```python
from build123d import *

# Parameters (mm, degrees)
F2_DEPTH = 105.9625
F3_W     = 176.60625
F3_H     = 3
F4_DEPTH = 6.35
F5_W     = 176.60625
F5_H     = 3
F6_DEPTH = 6.35


# Not quite as in the source:
# - a length typed as a fraction of an inch, garbled in the dataset ("3 / 203.2 mm" for 3/8 in), is restored


with BuildPart() as f2:
    # F1 (on Front) → F2 (new body)
    with BuildSketch(Plane.XZ):
        Polygon((-42.2606132925, -1.7798869123), (-42.2606132925, -4.7798869123), (134.3456367075, -4.7798869123), (134.3456367075, -1.7798869123), (127.9956367075, -1.7798869123), (127.9956367075, 1.2201130877), (-35.9106132925, 1.2201130877), (-35.9106132925, -1.7798869123), align=None)
    extrude(amount=F2_DEPTH)

    # F3 (on face) → F4 (join)
    with BuildSketch(Plane.XZ.offset(105.9625)):
        with Locations((46.0425117075, -3.2798869123)):
            Rectangle(F3_W, F3_H)
    extrude(amount=F4_DEPTH)

    # F5 (on face) → F6 (join)
    with BuildSketch(Plane(origin=(0, 0, 0), x_dir=(-1, 0, 0), z_dir=(0, 1, 0))):
        with Locations((-46.0425117075, -3.2798869123)):
            Rectangle(F5_W, F5_H)
    extrude(amount=F6_DEPTH)


solid = f2.part
```
Geometry check sheet. Reference: the model listing, model coordinates, mm. Give positions to 0.01 mm unless a question says otherwise; leave off trailing zeros. Write each loop counter-clockwise with the first axis right and the second up, starting at its lowest first coordinate (ties: lowest second). Pieces come first, ordered by that corner, then holes. Notation, with made-up numbers: (-25.75, 67) - (0.25, 67) arc R17 ccw to (0.25, 78) - close; hole circle Ø3 at (-37, -3.75). An arc over 180 degrees is marked (long way). Use a Markdown table: item, result.
Q1. Section check A-A, the plane x = 122.5. Enter the section's corners in (y, z).
Computed:
| item | result |
|---|---|
| outline | (-112.31, -4.78) - (6.35, -4.78) - (6.35, -1.78) - (0, -1.78) - (0, 1.22) - (-105.96, 1.22) - (-105.96, -1.78) - (-112.31, -1.78) - close |
Q2. Section check B-B, the plane y = -7. Enter the section's corners in (x, z), then the cut area to 3 significant figures.
Computed:
| item | result |
|---|---|
| outline | (-42.26, -4.78) - (134.35, -4.78) - (134.35, -1.78) - (128, -1.78) - (128, 1.22) - (-35.91, 1.22) - (-35.91, -1.78) - (-42.26, -1.78) - close |
| area | 1,020 mm² |
Q3. Thickness scan on L1, parallel to Z at x = 8, y = -106; L2, parallel to Y at x = 108, z = -0.65; L3, parallel to X at y = -3.5, z = -1.05. Record the ranges inside material, lowest first. Write a range as [from, to].
Computed:
| item | result |
|---|---|
| L1 | z = [-4.78, -1.78] |
| L2 | y = [-105.96, 0] |
| L3 | x = [-35.91, 128] |
Q4. Section check C-C, the plane z = 0.15. Enter the section's corners in (x, y).
Computed:
| item | result |
|---|---|
| outline | (-35.91, -105.96) - (128, -105.96) - (128, 0) - (-35.91, 0) - close |
Q5. Go/stop test with flat-tipped pins: P1, Ø2.5, axis at x = 22.5, z = 0, coming from the +Y side; P2, Ø1.5, axis at y = -38, z = -0.5, coming from the +X side; P3, Ø3.5, axis at x = 85.5, z = 0.5, coming from the -Y side. Record where each tip stops, or that it passes through.
Computed:
| item | result |
|---|---|
| P1 | stops at y = 0 |
| P2 | stops at x = 128 |
| P3 | stops at y = -105.96 |
